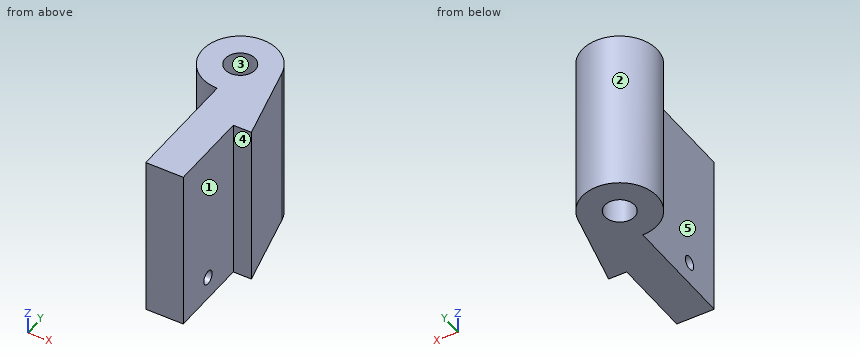
from build123d import *

# Parameters (mm, degrees)
ESQUISSE1_R             = 1.65
BOSS_EXTRU_1_DEPTH      = 9
ESQUISSE3_R             = 0.75
ENL_V_MAT_EXTRU_2_DEPTH = 21.949701669


with BuildPart() as part:
    # Esquisse1 → Boss.-Extru.1 (new, symmetric)
    with BuildSketch(Plane.XY):
        with BuildLine():
            Line((0, -4.15), (0, -17))
            Line((0, -17), (4.15, -17))
            Line((4.15, -17), (4.15, -8))
            Line((4.15, -8), (6.15, -8))
            Line((6.15, -8), (4.039246655, 0.952358366))
            ThreePointArc((4.039246655, 0.952358366), (-3.253827532, 2.575870026), (0, -4.15))
        make_face()
        Circle(ESQUISSE1_R, mode=Mode.SUBTRACT)
    extrude(amount=BOSS_EXTRU_1_DEPTH, both=True)

    # Esquisse3 → Enlèv. mat.-Extru.2 (cut, through all)
    with BuildSketch(Plane(origin=(4.15, 0, 0), x_dir=(0, 0, -1), z_dir=(1, 0, 0))):
        with Locations((6.46, -12.555)):
            Circle(ESQUISSE3_R)
    extrude(amount=-ENL_V_MAT_EXTRU_2_DEPTH, mode=Mode.SUBTRACT)


solid = part.part
Input: part model. Units: mm. Frame: model coordinates. Face numbers are marked on the shaded views. A direction names the side the tool comes from. Round coordinates to 2 decimals unless told otherwise and drop trailing zeros. Order: outer loops, then holes, each group sorted by start corner. A loop starts at its lowest first (then second) coordinate and runs counter-clockwise, first axis right, second up. Notation, with made-up numbers: (-10.5, 86.5) - (29.5, 86.5) arc R20 cw to (29.5, 116.5) - close; hole circle Ø8 at (69, 84.5). An arc over 180 degrees is marked (long way). Use a Markdown table: item, result.
1. Mould query, pull axis Y, two halves, no side actions, for the marked faces 3, 4 and 5. Classes: +Y half, -Y half, draft (parallel to the pull), parting line (faces both ways), or undercut.
Evaluation:
| item | result |
|---|---|
| face 3 | undercut |
| face 4 | -Y half |
| face 5 | draft |
2. Material intervals for probe 1 along X at (y, z) = (-15, 1.25); probe 2 along Y at (x, z) = (0.9, -6.46) (3 decimals); probe 3 along Y at (x, z) = (-0.5, 6.5), sorted ascending.
Evaluation:
| item | result |
|---|---|
| probe 1 | 0 to 4.15 |
| probe 2 | -17 to -13.305, -11.805 to -1.383, 1.383 to 4.051 |
| probe 3 | -4.12 to -1.57, 1.57 to 4.12 |
3. Section C-C on z = 5.5. Return the cut outline in (x, y), then the cut area to 3 significant figures.
Evaluation:
| item | result |
|---|---|
| outline | (0, -17) - (4.15, -17) - (4.15, -8) - (6.15, -8) - (4.04, 0.95) arc R4.15 ccw (long way) to (0, -4.15) - close; hole circle Ø3.3 at (0, 0) |
| area | 111 mm^2 |
4. Section A-A on z = -6.46. Return the cut outline in (x, y) (3 decimals), then the cut area to 3 significant figures.
Evaluation:
| item | result |
|---|---|
| outline | (0, -17) - (4.15, -17) - (4.15, -13.305) - (0, -13.305) - close; (0, -11.805) - (4.15, -11.805) - (4.15, -8) - (6.15, -8) - (4.039, 0.952) arc R4.15 ccw (long way) to (0, -4.15) - close; hole circle Ø3.3 at (0, 0) |
| area | 105 mm^2 |
5. Section D-D on x = -0.75. Return the cut outline in (y, z).
Evaluation:
| item | result |
|---|---|
| outline | (-4.08, -9) - (-1.47, -9) - (-1.47, 9) - (-4.08, 9) - close; (1.47, -9) - (4.08, -9) - (4.08, 9) - (1.47, 9) - close |
6. Access query for the marked faces 1 and 2. Directions: +Z, -Z, +X, -X, +Y, -Y. A direction counts if a zero-diameter tool reaches every point of the face in a straight line with its end or side. Return the directions, or none.
Evaluation:
| item | result |
|---|---|
| face 1 | +Z, -Z, +X, -Y |
| face 2 | +Z, -Z |
7. Section B-B on y = 0. Return the cut outline in (x, z), then the cut area to 3 significant figures.
Evaluation:
| item | result |
|---|---|
| outline | (-4.15, -9) - (-1.65, -9) - (-1.65, 9) - (-4.15, 9) - close; (1.65, -9) - (4.26, -9) - (4.26, 9) - (1.65, 9) - close |
| area | 92.0 mm^2 |
8. First-contact query: pin 1 (4 mm diameter, centred on x = 4, z = -4, fed in from +Y); pin 2 (6.5 mm diameter, centred on y = -8, z = 3.5, fed in from -X); pin 3 (1 mm diameter, centred on x = 4.5, z = -0.5, fed in from -Y); pin 4 (1.5 mm diameter, centred on y = -2, z = 2.5, fed in from +X). Flat tips, straight axial feed; report the tip coordinate or a pass-through.
Evaluation:
| item | result |
|---|---|
| pin 1 | y = 3.64 |
| pin 2 | x = 0 |
| pin 3 | y = -17 |
| pin 4 | x = 4.91 |
